Autodesk Inventor part; units mm, degrees
ref_plane "YZ Plane" through (0, 0, 0) normal (1, 0, 0) x (0, 1, 0)
ref_plane "XZ Plane" through (0, 0, 0) normal (0, 1, 0) x (-1, 0, 0)
ref_plane "XY Plane" through (0, 0, 0) normal (0, 0, 1) x (1, 0, 0)
sketch "Sketch1" plane through (0, 0, 0) normal (0, 0, 1) x (1, 0, 0)
  line L0 (0, 0) -> (0, 42.6644)
  line L1 (51.8018, 95.0115) -> (69.8, 95.2)
  arc A0 (51.8018, 95.0115) -> (0, 42.6644) centre (52.35, 42.6644) ccw
  dimension "d1" = 95.2
  dimension "d2" = 69.8
  dimension "d4" = 52.35
  dimension "d17" = 90.6
sketch "Sketch2" plane through (0, 0, 0) normal (0, 1, 0) x (-1, 0, 0)
  circle A0 centre (0, 0) radius 19.05
  circle A1 centre (0, 0) radius 17.4
  dimension "d3" = 38.1
  dimension "d11" = 1.65
sweep "Sweep1" add profiles "Sketch2" path "Sketch1"
sketch "Sketch3" plane through (69.8, 95.2, 0) normal (0.9999452, 0.0104718, 0) x (0, 0, -1)
  circle A0 centre (0, 0) radius 19.05
  circle A1 centre (0, 0) radius 25.15
  point P0 (0, -94.4638)
  dimension "d6" = 50.3
extrude "Extrusion1" add sketch "Sketch3" against normal blind 5
chamfer "Chamfer1" distance 3 distance2 3.8692 1 edges at (64.8003, 95.1476, 25.15) measured on face at (66.5091, 91.131, -24.8243)
equation "\"d4\" = 0.75 * d2"
equation "\"d15\" = 0.0769231 * d6"
properties part number "asme bpe - ferrule 90.6 deg elb-38.1"
Build history of the part. All positions in model axes, mm. Round coordinates to 2 decimals unless told otherwise and drop trailing zeros. Write each loop counter-clockwise with the first axis right and the second up, starting at its lowest first coordinate (ties: lowest second). Pieces come first, ordered by that corner, then holes. Notation, with made-up numbers: (33.5, 1) - (49.5, 1) arc R24 cw to (49.5, 38) - close; hole circle Ø6 at (-21.75, -30.75). An arc over 180 degrees is marked (long way). Write each question's results on one line, items separated by ' | '. Start each with the question number.
Item 1: Mould opens along X. For faces 1 (the face through (-15.43, 0, 8.38)), 2 (the face through (15.12, 21.63, -11.59)), 3 (the face through (64.92, 101.61, -20.53)), 4 (the face through (3.772, 21.631, -16.986)) say: pulls with the +X half, pulls with the -X half, needs draft (parallel to the pull), parting line crosses it, or undercut.
Item 2: Saw through at A-A (y = 24). Write the cut outline in (x, z), and give its area (3 significant figures).
Item 3: Wall check: L1, parallel to Z at x = 0, y = 31.5; L2, parallel to X at y = 40.5, z = -0.5; L3, parallel to Y at x = 18.5, z = 10.5. Give the ranges that are in metal, low to high. Write a range as [from, to].
Item 4: Drop flat-ended pins along their axis: P1, Ø4, axis at x = 37, z = -18, coming from the -Y side; P2, Ø4, axis at y = 71, z = -13.5, coming from the -X side; P3, Ø2, axis at x = 46.5, y = 76, coming from the +Z side. Give the stop position or say it passes through.
Results are:
1) face 1: needs draft | face 2: parting line crosses it | face 3: undercut | face 4: undercut
2) outline: circle Ø38.1 at (0, 0); hole circle Ø34.8 at (0, 0) | area: 189 mm²
3) L1: z = [-19.05, -17.4], [17.4, 19.05] | L2: x = [-19.04, -17.39], [17.39, 19.04] | L3: y = [56.2, 60.95], [99.58, 101.92]
4) P1: stops at y = 81.68 | P2: stops at x = -9.18 | P3: stops at z = 7.52
